```python
from build123d import *

# Parameters (mm, degrees)
BOX002_W       = 90
BOX002_H       = 90
BOX002_DEPTH   = 3.4
ARRAY004_COUNT = 3
ARRAY004_ANGLE = 180
ARRAY_COUNT    = 4
BOX_W          = 16
BOX_H          = 16
BOX_DEPTH      = 16


with BuildPart() as array:
    # Box002 → Box002 (new body)
    with BuildSketch(Plane(origin=(3, 3, -1.7), x_dir=(1, 0, 0), z_dir=(0, 0, 1))):
        with Locations((45, 45)):
            Rectangle(BOX002_W, BOX002_H)
    extrude(amount=BOX002_DEPTH)

    # Array004: Array ×3 about axis
    array004_axis = Axis((0, 0, 0), (0, 1, 0))


with BuildPart() as array_1:
    add(array.part)
    for i in range(1, ARRAY004_COUNT):
        add(array.part.rotate(array004_axis, i * ARRAY004_ANGLE / (ARRAY004_COUNT - 1)))

    # Array: Array ×4 about axis
    array_axis = Axis((0, 0, 0), (1, 0, 0))


with BuildPart() as array_2:
    add(array_1.part)
    for i in range(1, ARRAY_COUNT):
        add(array_1.part.rotate(array_axis, i * 360 / ARRAY_COUNT))


with BuildPart() as cut001:
    # Box → Box (new body)
    with BuildSketch(Plane(origin=(-8, -8, -8), x_dir=(1, 0, 0), z_dir=(0, 0, 1))):
        with Locations((8, 8)):
            Rectangle(BOX_W, BOX_H)
    extrude(amount=BOX_DEPTH)

    # Cut001: cut Array
    add(array_2.part, mode=Mode.SUBTRACT)


solid = cut001.part
```
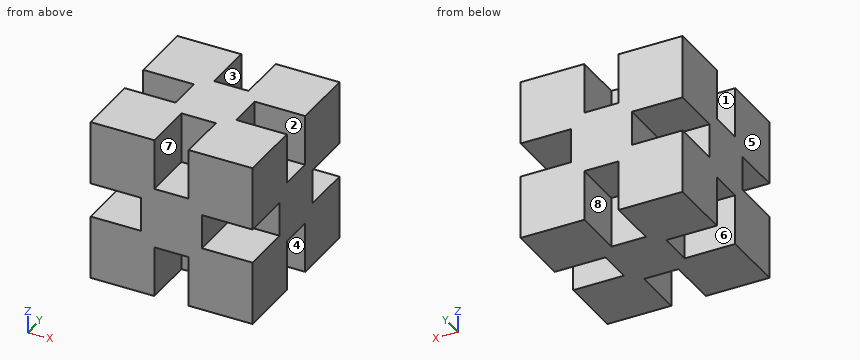
Input: part model. Units: mm. Frame: model coordinates. Face numbers are marked on the shaded views. A direction names the side the tool comes from. Give positions to 0.01 mm unless a question says otherwise; leave off trailing zeros. Write each loop counter-clockwise with the first axis right and the second up, starting at its lowest first coordinate (ties: lowest second). Pieces come first, ordered by that corner, then holes. Notation, with made-up numbers: (25, 82.25) - (50, 82.25) arc R21 cw to (50, 94.25) - close; hole circle Ø2 at (33.25, 23.5). An arc over 180 degrees is marked (long way). Write item = value, one per line. Start each with the question number.
1. Section query B-B, the plane z = 1.25. Output: boundary loops of the cut face in (x, y).
2. Section query A-A, the plane x = -5.5. Output: boundary loops of the cut face in (y, z), then the cut area to 3 significant figures.
3. Access query for the marked faces 1, 2, 3 and 4. Directions: +Z, -Z, +X, -X, +Y, -Y. A direction counts if a zero-diameter tool reaches every point of the face in a straight line with its end or side. Return the directions, or none.
4. Ray query, L1, parallel to Z at x = -6, y = -4. Return the intervals inside material, ascending.
5. Mould query, pull axis X, two halves, no side actions, for the marked faces 5, 6, 7 and 8. Classes: released by +X, released by -X, zero draft, split by the parting line, or undercut.
6. First-contact query: pin 1 Ø1 at (x, z) = (-6, -0.5) entering from +Y. Flat tip, straight axial feed; report the tip coordinate or a pass-through.
Check sheet entries:
q1.outline = (-8, -3) - (-3, -3) - (-3, -8) - (3, -8) - (3, -3) - (8, -3) - (8, 3) - (3, 3) - (3, 8) - (-3, 8) - (-3, 3) - (-8, 3) - close
q2.outline = (-8, -8) - (-1.7, -8) - (-1.7, -3) - (1.7, -3) - (1.7, -8) - (8, -8) - (8, -1.7) - (3, -1.7) - (3, 1.7) - (8, 1.7) - (8, 8) - (1.7, 8) - (1.7, 3) - (-1.7, 3) - (-1.7, 8) - (-8, 8) - (-8, 1.7) - (-3, 1.7) - (-3, -1.7) - (-8, -1.7) - close
q2.area = 188 mm2
q3.face_1 = +Z, -X
q3.face_2 = +Z, +X
q3.face_3 = +Z, +Y
q3.face_4 = -Z, +X
q4.L1 = -8 to -1.7, 1.7 to 8
q5.face_5 = released by -X
q5.face_6 = zero draft
q5.face_7 = undercut
q5.face_8 = undercut
q6.pin_1 = 3
